Check sheet for the drawn part. Datum: minimum x, y, z corner. Units: mm. A direction names the side the tool comes from. Give positions to 0.01 mm unless a question says otherwise; leave off trailing zeros. Order: outer loops, then holes, each group sorted by start corner. A loop starts at its lowest first (then second) coordinate and runs counter-clockwise, first axis right, second up. Notation, with made-up numbers: (13.25, 80) - (27.25, 80) arc R35 cw to (27.25, 112) - close; hole circle Ø6 at (17, 18). An arc over 180 degrees is marked (long way). Answer as a JSON object with one key per item and string values. Group by question number.
(1) Section check A-A (x = 36). Record the boundary of the cut face in (y, z), then the cut area to 3 significant figures.
(2) Section check B-B (z = 29.5). Record the boundary of the cut face in (x, y).
(3) Depth check by flat-ended pin: pin 1 Ø19 at (x, y) = (57, 63.5) entering from +Z; pin 2 Ø4 at (x, y) = (79.5, 44) entering from +Z; pin 3 Ø17 at (y, z) = (24, 37.5) entering from +X. Enter the tip coordinate at first touch or a pass-through.
(4) Section check C-C (y = 49). Record the boundary of the cut face in (x, z).
(5) Access from +Z, -Z, +X, -X, +Y, -Y to the whole of each face (thin tool, end or side, straight path). Record for the marked faces 5, 6 and 7.
(6) Thickness scan on line 1 (Y direction, x = 36, z = 16.5); line 2 (Z direction, x = 11, y = 40.5); line 3 (Y direction, x = 30.5, z = 19.5) (1 decimal). Record the ranges inside material, lowest first.
(7) Mould release check, pull along Z, two halves, no side actions. Record for the marked faces 1, 2, 3 and 4: +Z half, -Z half, draft (parallel to the pull), parting line (faces both ways), or undercut.
(8) Section check D-D (z = 63). Record the boundary of the cut face in (x, y) (1 decimal), then the cut area to 3 significant figures.
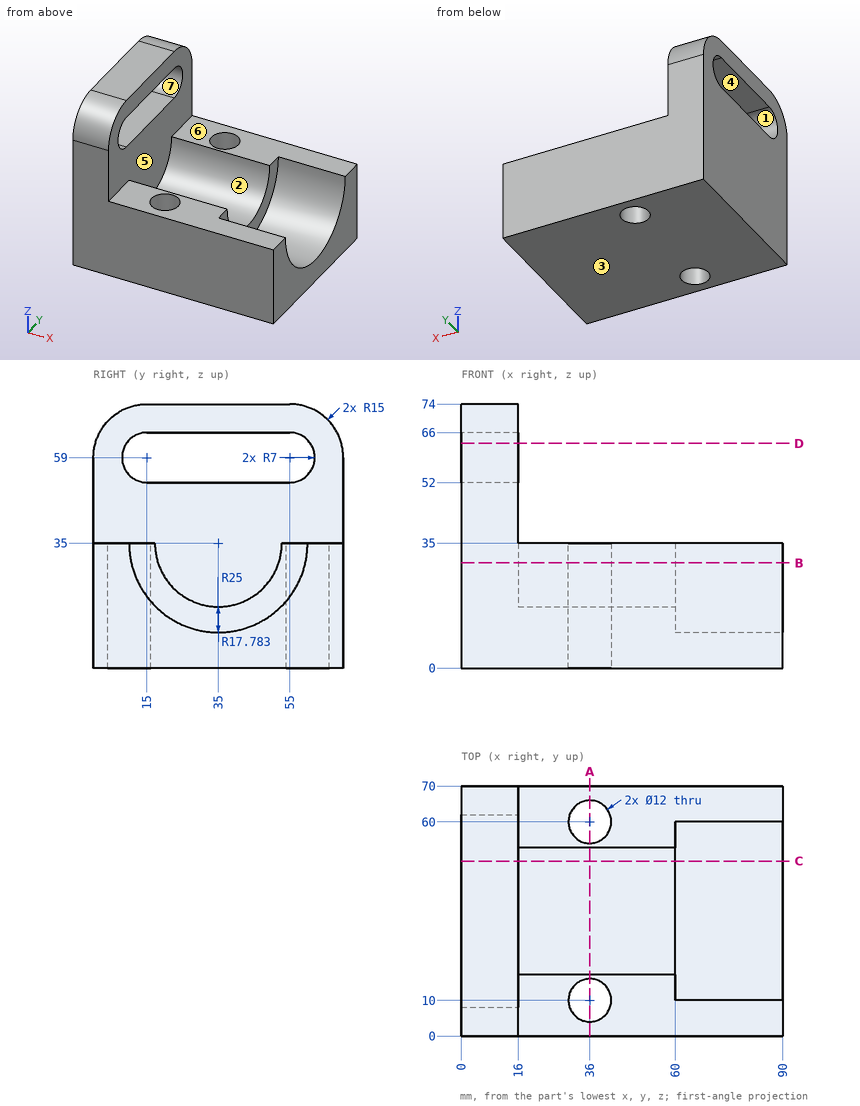
Solutions:
{
 "1": {"outline": "(0, 0) - (4, 0) - (4, 35) - (0, 35) - close; (16, 0) - (54, 0) - (54, 35) - (52.78, 35) arc R17.78 cw to (17.22, 35) - (16, 35) - close; (66, 0) - (70, 0) - (70, 35) - (66, 35) - close", "area": "1,110 mm2"},
 "2": {"outline": "(0, 0) - (90, 0) - (90, 10.61) - (60, 10.61) - (60, 18.09) - (16, 18.09) - (16, 51.91) - (60, 51.91) - (60, 59.39) - (90, 59.39) - (90, 70) - (0, 70) - close; hole circle Ø12 at (36, 10); hole circle Ø12 at (36, 60)"},
 "3": {"pin 1": "stops at z = 35", "pin 2": "stops at z = 12.55", "pin 3": "stops at x = 60"},
 "4": {"outline": "(0, 0) - (90, 0) - (90, 14.29) - (60, 14.29) - (60, 24.03) - (16, 24.03) - (16, 52) - (0, 52) - close; (0, 66) - (16, 66) - (16, 74) - (0, 74) - close"},
 "5": {"face 5": "+Z, +X", "face 6": "+Z, +X, +Y, -Y", "face 7": "+X, -X"},
 "6": {"line 1": "y = 0 to 4, 16 to 54, 66 to 70", "line 2": "z = 0 to 52, 66 to 74", "line 3": "y = 0 to 7.6, 12.4 to 26.3, 43.7 to 57.6, 62.4 to 70"},
 "7": {"face 1": "undercut", "face 2": "+Z half", "face 3": "-Z half", "face 4": "undercut"},
 "8": {"outline": "(0, 0.5) - (16, 0.5) - (16, 9.3) - (0, 9.3) - close; (0, 60.7) - (16, 60.7) - (16, 69.5) - (0, 69.5) - close", "area": "279 mm2"}
}
